Design review of the part built by this model. Coordinates are the model's own, in mm. A direction names the side the tool comes from. Give positions to 0.01 mm unless a question says otherwise; leave off trailing zeros. Order: outer loops, then holes, each group sorted by start corner. A loop starts at its lowest first (then second) coordinate and runs counter-clockwise, first axis right, second up. Notation, with made-up numbers: M -37.75,26.25 L -21.75,26.25 A24 ccw -21.75,62.25 Z; hole C 10.25,26.5 d10. An arc over 180 degrees is marked long. Put each result on its own line as item: value. Start each with the question number.
from build123d import *

# Parameters (mm, degrees)
SKETCH3_R      = 5
EXTRUDE2_DEPTH = 20
SKETCH2_R      = 5
EXTRUDE3_DEPTH = 20


with BuildPart() as part:
    # Sketch1 → Revolve1 (revolve)
    with BuildSketch(Plane.XY, mode=Mode.PRIVATE) as revolve1_sk:
        with BuildLine():
            Line((-89.926247849, 0), (-89.926247849, 13.5))
            ThreePointArc((-89.926247849, 13.5), (-89.194014801, 15.267766953), (-87.426247849, 16))
            Line((-87.426247849, 16), (-53.926247849, 16))
            Line((-53.926247849, 16), (-53.926247849, 10))
            Line((-53.926247849, 10), (155.073752151, 10))
            Line((155.073752151, 10), (155.073752151, 6))
            Line((155.073752151, 6), (172.073752151, 6))
            Line((172.073752151, 6), (172.073752151, 5))
            Line((172.073752151, 5), (190.073752151, 5))
            Line((190.073752151, 5), (190.073752151, 0))
            Line((190.073752151, 0), (-89.926247849, 0))
        make_face()
    revolve(revolve1_sk.sketch.rotate(Axis((0, 0, 0), (1, 0, 0)), 90), axis=Axis((0, 0, 0), (1, 0, 0)))

    # Sketch3 → Extrude2 (cut, symmetric)
    with BuildSketch(Plane.XY):
        with Locations((-71.926247849, 0)):
            Circle(SKETCH3_R)
    extrude(amount=EXTRUDE2_DEPTH, both=True, mode=Mode.SUBTRACT)

    # Sketch2 → Extrude3 (cut, symmetric)
    with BuildSketch(Plane(origin=(0, 0, 0), x_dir=(1, 0, 0), z_dir=(0, 1, 0))):
        with Locations(Location((-71.926247849, 0, 0), (0, 0, 270))):
            Circle(SKETCH2_R)
    extrude(amount=EXTRUDE3_DEPTH, both=True, mode=Mode.SUBTRACT)


solid = part.part
1. Consider section A-A on x = 61.5. Give the boundary of the cut face in (y, z).
2. To check wall thickness, follow probe 1 along X at (y, z) = (0, -12); probe 2 along X at (y, z) = (0, -5.5); probe 3 along X at (y, z) = (-7, 12). State the ranges of each line that lie inside material, in increasing order.
3. Insertion check: pin 1 (8 mm diameter, centred on x = 123.5, y = -8, fed in from +Z); pin 2 (8 mm diameter, centred on x = -71.93, z = 0, fed in from +Y); pin 3 (1 mm diameter, centred on x = 116, y = 5, fed in from +Z); pin 4 (5 mm diameter, centred on x = 47.5, y = -10, fed in from +Z). Each pin has a flat end and moves straight along its axis. Give the tip position at first contact, or say it passes through.
4. Machinability: for faces 1 (the cylindrical face through (52, 0, -10)), 2 (the flat face through (190.074, 0, 0)), which of the approach directions +Z, -Z, +X, -X, +Y, -Y give a long, thin tool a straight path to every point of the face, cutting with its end or side? Answer none if there is none.
5. The part is to be moulded in two halves that separate along X. For faces 3 (the cylindrical face through (-67.71, 9.89, 2.69)), 4 (the cylindrical face through (163.693, -1.802, 5.723)), 5 (the flat face through (155.074, 0, 7)), say which applies: +X half, -X half, draft (parallel to the pull), parting line (faces both ways), or undercut.
Returned:
1. outline: C 0,0 d20
2. probe 1: x = -89.93 to -76.93, -66.93 to -53.93
2. probe 2: x = -89.93 to -76.93, -66.93 to 172.07
2. probe 3: x = -89.9 to -53.93
3. pin 1: stops at z = 9.17
3. pin 2: passes through
3. pin 3: stops at z = 8.93
3. pin 4: stops at z = 6.61
4. face 1: +X
4. face 2: +Z, -Z, +X, +Y, -Y
5. face 3: undercut
5. face 4: draft
5. face 5: +X half
